The figure shows three views and two pictorial views of one solid part (mm, origin at its lowest corner). Answer the questions. A direction names the side the tool comes from. Round coordinates to 2 decimals unless told otherwise and drop trailing zeros. Order: outer loops, then holes, each group sorted by start corner. A loop starts at its lowest first (then second) coordinate and runs counter-clockwise, first axis right, second up. Notation, with made-up numbers: M -22.75,-1 L 17.25,-1 A25 ccw 17.25,27 Z; hole C 63,-32 d3. An arc over 180 degrees is marked long. Return JSON: item names as keys, results as strings.
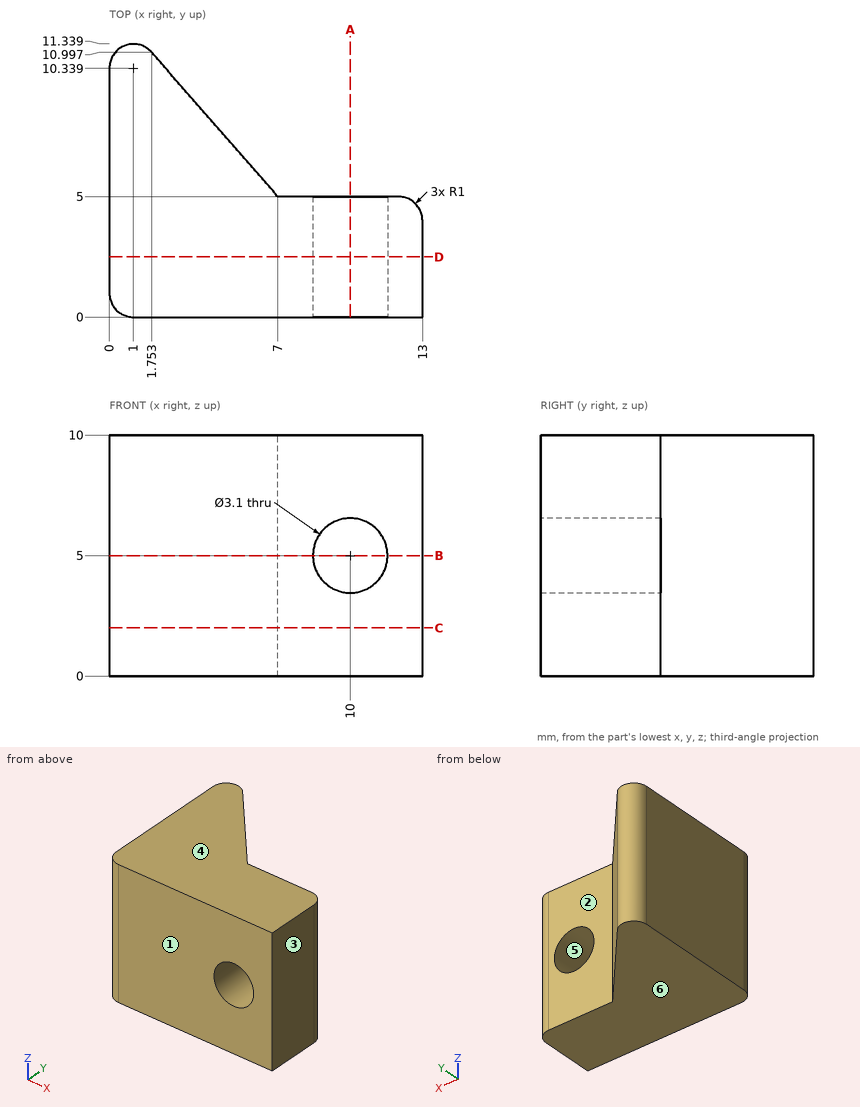
Item 1: Which of the six approach directions +Z, -Z, +X, -X, +Y, -Y give full straight-line access (tool end or side, diameter ignored) to the marked faces 1 and 2?
Output:
{"face 1": "+Z, -Z, +X, -X, -Y", "face 2": "+Z, -Z, +X, +Y"}
Item 2: Find section A-A (x = 10). Determine the outline of the cut face in (y, z), plus the area to 3 significant figures.
Output:
{"outline": "M 0,0 L 5,0 L 5,3.45 L 0,3.45 Z; M 0,6.55 L 5,6.55 L 5,10 L 0,10 Z", "area": "34.5 mm^2"}
Item 3: Find section B-B (z = 5). Determine the outline of the cut face in (x, y).
Output:
{"outline": "M 0,1 A1 ccw 1,0 L 8.45,0 L 8.45,5 L 7,5 L 1.75,11 A1 ccw 0,10.34 Z; M 11.55,0 L 13,0 L 13,4 A1 ccw 12,5 L 11.55,5 Z"}
Item 4: Find section D-D (y = 2.5). Determine the outline of the cut face in (x, z).
Output:
{"outline": "M 0,0 L 13,0 L 13,10 L 0,10 Z; hole C 10,5 d3.1"}
Item 5: Each of these flat-tipped pins is pushed along its axis until it touches: pin 1 (4 mm diameter, centred on x = 10, z = 5, fed in from -Y); pin 2 (5.5 mm diameter, centred on x = 8.5, z = 6, fed in from +Y). Where does it stop, or does it pass through?
Output:
{"pin 1": "stops at y = 0", "pin 2": "stops at y = 6.43"}
Item 6: Consider line 1 along X through (y, z) = (3.85, 5); line 2 along Y through (x, z) = (10, 8.25); line 3 along Y through (x, z) = (5.25, 7.5). Determine where each line is inside the solid, lowest interval first. Write a range as [from, to].
Output:
{"line 1": "x = [0, 8.45], [11.55, 13]", "line 2": "y = [0, 5]", "line 3": "y = [0, 7]"}
Item 7: Find section C-C (z = 2). Determine the outline of the cut face in (x, y).
Output:
{"outline": "M 0,1 A1 ccw 1,0 L 13,0 L 13,4 A1 ccw 12,5 L 7,5 L 1.75,11 A1 ccw 0,10.34 Z"}
Item 8: The mould has two halves that part along Z. Classify the marked faces 3, 4, 5 and 6: pulls with the +Z half, pulls with the -Z half, needs draft (parallel to the pull), parting line crosses it, or undercut.
Output:
{"face 3": "needs draft", "face 4": "pulls with the +Z half", "face 5": "undercut", "face 6": "pulls with the -Z half"}
